CAD build for the part. Positions are in the model's coordinates, mm. Face numbers are marked on the shaded views. A direction names the side the tool comes from. Coordinates: 2 decimals unless noted, no trailing zeros. Write each loop counter-clockwise with the first axis right and the second up, starting at its lowest first coordinate (ties: lowest second). Pieces come first, ordered by that corner, then holes. Notation, with made-up numbers: (26.25, -33) -> (71.25, -33) arc R27 cw to (71.25, -6) -> close; hole circle Ø1 at (22, -19). An arc over 180 degrees is marked (long way). Answer as CSV lines item,"result".
```python
from build123d import *

# Parameters (mm, degrees)
BOSS_EXTRUDE1_DEPTH = 20
SKETCH3_R           = 1.5
CUT_EXTRUDE1_DEPTH  = 3
FILLET1_R           = 1


with BuildPart() as part:
    # Sketch2 → Boss-Extrude1 (new body)
    with BuildSketch(Plane.XY):
        Polygon((-20.25, 19), (20.25, 19), (20.25, 0), (32.25, 0), (32.25, 2), (22.25, 2), (22.25, 21), (-22.25, 21), (-22.25, 2), (-32.25, 2), (-32.25, 0), (-20.25, 0), align=None)
    extrude(amount=BOSS_EXTRUDE1_DEPTH)

    # Sketch3 → Cut-Extrude1 (cut, through all)
    with BuildSketch(Plane(origin=(0, 2, 0), x_dir=(1, 0, 0), z_dir=(0, 1, 0))):
        with Locations((27.25, -6)):
            Circle(SKETCH3_R)
        with Locations((27.25, -14)):
            Circle(SKETCH3_R)
        with Locations((-27.25, -14)):
            Circle(SKETCH3_R)
        with Locations((-27.25, -6)):
            Circle(SKETCH3_R)
    extrude(amount=-CUT_EXTRUDE1_DEPTH, mode=Mode.SUBTRACT)

    # Fillet1
    fillet1_edges = [part.edges().sort_by_distance(p)[0] for p in [
        (-22.25, 2, 10),
        (-22.25, 21, 10),
        (22.25, 21, 10),
        (22.25, 2, 10),
    ]]
    fillet(fillet1_edges, radius=FILLET1_R)


solid = part.part
```
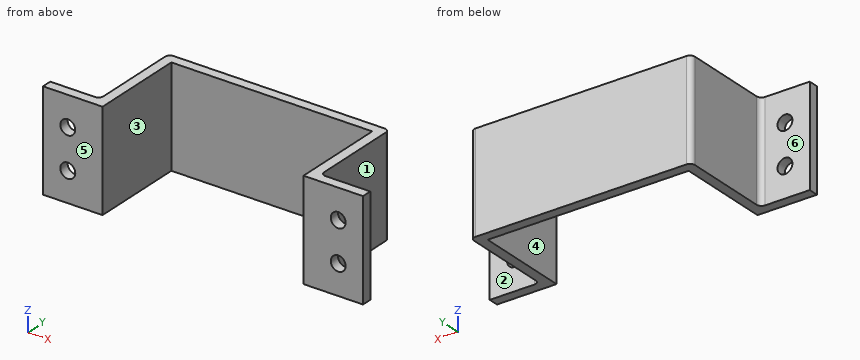
Item 1: Saw through at A-A on y = 18. Give the cut face in (x, z), and give its area (3 significant figures).
Answer below:
outline,"(-22.25, 0) -> (-20.25, 0) -> (-20.25, 20) -> (-22.25, 20) -> close; (20.25, 0) -> (22.25, 0) -> (22.25, 20) -> (20.25, 20) -> close"
area,"80.0 mm2"
Item 2: Flat gauge pins, fed straight in: pin 1 (2.5 mm diameter, centred on x = 27.25, z = 14, fed in from -Y); pin 2 (1.5 mm diameter, centred on y = 6, z = 17.5, fed in from +X); pin 3 (5.5 mm diameter, centred on y = 14, z = 7.5, fed in from -X); pin 4 (10 mm diameter, centred on x = -29, z = 13.5, fed in from +Y). Where does each tip first touch, or does it go through?
Answer below:
pin 1,"passes through"
pin 2,"stops at x = 22.25"
pin 3,"stops at x = -22.25"
pin 4,"stops at y = 2"
Item 3: Saw through at B-B on z = 6. Give the cut face in (x, y), and give its area (3 significant figures).
Answer below:
outline,"(-32.25, 0) -> (-28.75, 0) -> (-28.75, 2) -> (-32.25, 2) -> close; (-25.75, 0) -> (-20.25, 0) -> (-20.25, 19) -> (20.25, 19) -> (20.25, 0) -> (25.75, 0) -> (25.75, 2) -> (23.25, 2) arc R1 cw to (22.25, 3) -> (22.25, 20) arc R1 ccw to (21.25, 21) -> (-21.25, 21) arc R1 ccw to (-22.25, 20) -> (-22.25, 3) arc R1 cw to (-23.25, 2) -> (-25.75, 2) -> close; (28.75, 0) -> (32.25, 0) -> (32.25, 2) -> (28.75, 2) -> close"
area,"193 mm2"
Item 4: Wall check: line 1 (Z direction, x = -27.25, y = 1.2); line 2 (X direction, y = 7, z = 6.75); line 3 (X direction, y = 1.35, z = 6). Give the ranges that are in metal, low to high. Write a range as from..to.
Answer below:
line 1,"z = 0..4.5, 7.5..12.5, 15.5..20"
line 2,"x = -22.25..-20.25, 20.25..22.25"
line 3,"x = -32.25..-28.75, -25.75..-20.25, 20.25..25.75, 28.75..32.25"
Item 5: Saw through at D-D on z = 8.75. Give the cut face in (x, y), and give its area (3 significant figures).
Answer below:
outline,"(-32.25, 0) -> (-20.25, 0) -> (-20.25, 19) -> (20.25, 19) -> (20.25, 0) -> (32.25, 0) -> (32.25, 2) -> (23.25, 2) arc R1 cw to (22.25, 3) -> (22.25, 20) arc R1 ccw to (21.25, 21) -> (-21.25, 21) arc R1 ccw to (-22.25, 20) -> (-22.25, 3) arc R1 cw to (-23.25, 2) -> (-32.25, 2) -> close"
area,"205 mm2"
Item 6: Two-plate mould, pull along X, no slides. Class the marked faces 1, 2 and 3: pulls with the +X half, pulls with the -X half, needs draft (parallel to the pull), parting line crosses it, or undercut.
Answer below:
face 1,"pulls with the +X half"
face 2,"needs draft"
face 3,"undercut"
Item 7: 3-axis set-ups, long thin cutter, end or side, ignore diameter. For the marked faces 4, 5 and 6: which of +Z, -Z, +X, -X, +Y, -Y reach the whole face in a straight line?
Answer below:
face 4,"+Z, -Z, -Y"
face 5,"+Z, -Z, +X, -X, -Y"
face 6,"+Z, -Z, -X, +Y"
Item 8: Saw through at C-C on x = 27.25. Give the cut face in (y, z).
Answer below:
outline,"(0, 0) -> (2, 0) -> (2, 4.5) -> (0, 4.5) -> close; (0, 7.5) -> (2, 7.5) -> (2, 12.5) -> (0, 12.5) -> close; (0, 15.5) -> (2, 15.5) -> (2, 20) -> (0, 20) -> close"
